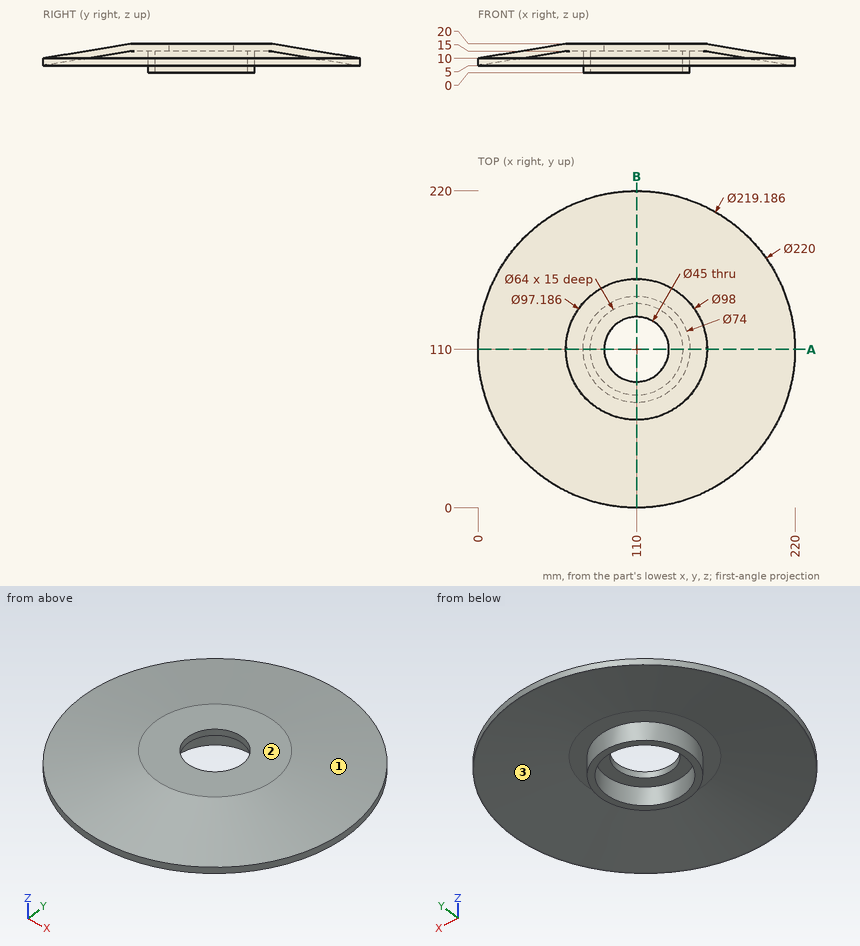
The drawing under review shows one solid part. Ordinate dimensions are in mm from its lowest x, y, z. Round coordinates to 2 decimals unless told otherwise and drop trailing zeros. Loops run counter-clockwise (first coordinate to the right, second up) from the corner with the lowest first, then second, coordinate; pieces in that order, holes last. Notation, with made-up numbers: (-14, 19) - (30, 19) arc R26 cw to (30, 46) - close; hole circle Ø10 at (23.25, 53.25). An arc over 180 degrees is marked (long way). Use a Markdown table: item, result. Add a question column.
Q1. Add section A-A (y = 110). State the section outline as (x, z) points, plus the area to 3 significant figures.
Q2. The part is to be moulded in two halves that separate along X. For the marked faces 1, 2 and 3, say which applies: pulls with the +X half, pulls with the -X half, needs draft (parallel to the pull), parting line crosses it, or undercut.
Q3. For probe 1 along Y at (x, z) = (82.5, 2.25) (1 decimal); probe 2 along Z at (x, y) = (98, 145.5); probe 3 along Z at (x, y) = (98, 204), list the stretches that pass through material, from the lowest coordinate up.
Q4. Insertion check: pin 1 Ø1.5 at (y, z) = (139.5, 9.5) entering from +X; pin 2 Ø1.5 at (x, z) = (130, 3.5) entering from +Y; pin 3 Ø6 at (x, y) = (173, 160) entering from -Z. Each pin has a flat end and moves straight along its axis. Give the tip position at first contact, or say it passes through.
Worked answers:
| question | item | result |
|---|---|---|
| 1 | outline | (0, 5) - (0.41, 5) - (61.41, 15) - (73, 15) - (73, 0) - (78, 0) - (78, 15) - (87.5, 15) - (87.5, 20) - (61, 20) - (0, 10) - close; (132.5, 15) - (142, 15) - (142, 0) - (147, 0) - (147, 15) - (158.59, 15) - (219.59, 5) - (220, 5) - (220, 10) - (159, 20) - (132.5, 20) - close |
| 1 | area | 1,030 mm² |
| 2 | face 1 | parting line crosses it |
| 2 | face 2 | needs draft |
| 2 | face 3 | undercut |
| 3 | probe 1 | 85.2 to 93.6, 126.4 to 134.8 |
| 3 | probe 2 | 15 to 20 |
| 3 | probe 3 | 7.43 to 12.5 |
| 4 | pin 1 | x = 216.18 |
| 4 | pin 2 | y = 141.6 |
| 4 | pin 3 | z = 9.29 |
